Part model, mm, in its own coordinate system. A direction names the side the tool comes from. Round coordinates to 2 decimals unless told otherwise and drop trailing zeros. Loops run counter-clockwise (first coordinate to the right, second up) from the corner with the lowest first, then second, coordinate; pieces in that order, holes last. Notation, with made-up numbers: (76, 15.5) - (103, 15.5) arc R12 ccw to (103, 33.5) - close; hole circle Ø9 at (52, 6). An arc over 180 degrees is marked (long way). Write each question's results on one line, items separated by ' | '. Start each with the question number.
(1) Drill centre lines: L1, parallel to Y at x = -76.5, z = 2.7; L2, parallel to Y at x = -60, z = 2.7; L3, parallel to X at y = -9.5, z = 0.7. Where is each one in solid material? Low to high.
(2) Cut at B-B, the plane z = 1.3. List the corners of the cut face in (x, y).
(3) Mould opens along Y. For faces 1 (the face through (-114.985, 1.826, 1.972)), 2 (the face through (-50.744, 108.82, 0.986)), 3 (the face through (-115, 6, 0)) say: released by +Y, released by -Y, zero draft, split by the parting line, or undercut.
(4) Cut at A-A, the plane x = -84.5. List the corners of the cut face in (y, z).
(5) Tool access for faces 4 (the face through (-68.9, 98.4, 3)), 5 (the face through (-50.685, -108.693, 2.986)), 6 (the face through (-68.79, -98.24, 0.99)): list every direction of +Z, -Z, +X, -X, +Y, -Y with a clear straight run to the whole face (end or side of a thin tool).
(6) Cut at D-D, the plane y = 32.5. List the corners of the cut face in (x, z).
(7) Cut at C-C, the plane y = 76.5. List the corners of the cut face in (x, z), then the cut area to 3 significant figures.
(8) Flat gauge pins, fed straight in: P1, Ø21, axis at x = -59, y = 108, coming from the +Z side; P2, Ø1.5, axis at x = -63, z = 3.5, coming from the -Y side; P3, Ø3, axis at x = -60, y = -103.92, coming from the -Z side; P4, Ø5.5, axis at x = -63.5, y = -99, coming from the -Z side. Where does each tip first touch, or does it go through?
from build123d import *

# Parameters (mm, degrees)
BOSS_EXTRU_1_DEPTH      = 4
ESQUISSE3_R             = 1.75
ENL_V_MAT_EXTRU_1_DEPTH = 10
ENL_V_START             = -2
ENL_V_MAT_EXTRU_2_DEPTH = 2
ENL_V_MAT_EXTRU_3_DEPTH = 2


with BuildPart() as part:
    # Esquisse1 → Boss.-Extru.1 (new body)
    with BuildSketch(Plane.XY):
        with BuildLine():
            Line((-48.6011001, -104.225395509), (-52.827282718, -113.28847338))
            ThreePointArc((-52.827282718, -113.28847338), (-105.423930727, -67.162451043), (-125, 0))
            ThreePointArc((-125, 0), (-105.423930727, 67.162451043), (-52.827282718, 113.28847338))
            Line((-52.827282718, 113.28847338), (-48.6011001, 104.225395509))
            ThreePointArc((-48.6011001, 104.225395509), (-115, 0), (-48.6011001, -104.225395509))
        make_face()
    extrude(amount=BOSS_EXTRU_1_DEPTH)

    # Esquisse3 → Enlèv. mat.-Extru.1 (cut)
    with BuildSketch(Plane.XY.offset(4)):
        with Locations((-60, 103.923048454)):
            Circle(ESQUISSE3_R)
        with Locations((-60, -103.923048454)):
            Circle(ESQUISSE3_R)
    extrude(amount=-ENL_V_MAT_EXTRU_1_DEPTH, mode=Mode.SUBTRACT)

    # Esquisse4 → Enlèv. mat.-Extru.2 (cut)
    with BuildSketch(Plane.XY.offset(4).offset(ENL_V_START)):
        with BuildLine():
            Line((-71.697054544, 102.394005536), (-65.96129018, 94.202485093))
            ThreePointArc((-65.96129018, 94.202485093), (-57.5, 99.592921435), (-48.6011001, 104.225395509))
            Line((-48.6011001, 104.225395509), (-52.827282718, 113.28847338))
            ThreePointArc((-52.827282718, 113.28847338), (-62.5, 108.253175473), (-71.697054544, 102.394005536))
        make_face()
    extrude(amount=ENL_V_MAT_EXTRU_2_DEPTH, mode=Mode.SUBTRACT)

    # Esquisse6 → Enlèv. mat.-Extru.3 (cut)
    with BuildSketch(Plane(origin=(0, 0, 0), x_dir=(-1, 0, 0), z_dir=(0, 0, -1))):
        with BuildLine():
            Line((65.96129018, -94.202485093), (71.697054544, -102.394005536))
            ThreePointArc((71.697054544, -102.394005536), (62.5, -108.253175473), (52.827282718, -113.28847338))
            Line((52.827282718, -113.28847338), (48.6011001, -104.225395509))
            ThreePointArc((48.6011001, -104.225395509), (57.5, -99.592921435), (65.96129018, -94.202485093))
        make_face()
    extrude(amount=-ENL_V_MAT_EXTRU_3_DEPTH, mode=Mode.SUBTRACT)


solid = part.part
A:
1) L1: -98.86 to -85.86, 85.86 to 98.86 | L2: -109.66 to -105.67, -102.17 to -98.11 | L3: -124.64 to -114.61
2) outline: (-71.7, -102.39) - (-65.96, -94.2) arc R115 cw to (-48.6, 104.23) - (-52.83, 113.29) arc R125 ccw to start; hole circle Ø3.5 at (-60, 103.92)
3) face 1: undercut | face 2: released by +Y | face 3: zero draft
4) outline: (-92.11, 0) - (-78, 0) - (-78, 4) - (-92.11, 4) - close; (78, 0) - (92.11, 0) - (92.11, 4) - (78, 4) - close
5) face 4: +Z, +X, +Y | face 5: +Z, -Z, +X, -Y | face 6: -Z, +X, -Y
6) outline: (-120.7, 0) - (-110.31, 0) - (-110.31, 4) - (-120.7, 4) - close
7) outline: (-98.86, 0) - (-85.86, 0) - (-85.86, 4) - (-98.86, 4) - close | area: 52.0 mm2
8) P1: z = 2 | P2: y = -108.4 | P3: through | P4: z = 2
